Model file for the job. Use its own axes, mm. Face numbers are marked on the shaded views. Coordinates: 2 decimals unless noted, no trailing zeros. Write each loop counter-clockwise with the first axis right and the second up, starting at its lowest first coordinate (ties: lowest second). Pieces come first, ordered by that corner, then holes.
Q1. Band-saw the part on C-C, the plane z = 9.25. Write the cut outline in (x, y) (3 decimals).
Q2. Band-saw the part on B-B, the plane y = 25. Write the cut outline in (x, z).
Q3. Band-saw the part on A-A, the plane x = 0. Write the cut outline in (y, z) (3 decimals).
Q4. Drill centre lines: probe 1 along X at (y, z) = (0.5, 4.25); probe 2 along Y at (x, z) = (-23, 5.5); probe 3 along X at (y, z) = (-12, 0.75). Where is each one in solid material? Low to high.
Q5. Pin check, flat tips, straight feed: P1, Ø1, axis at x = -20.5, z = 3.5, coming from the -Y side; P2, Ø1.5, axis at x = -0.5, z = 7, coming from the -Y side; P3, Ø6, axis at x = -5, z = 6, coming from the -Y side. Stop position of each tip, or through.
Q6. Pull direction X, two halves, no side cores. Call the marked faces 1, 2 and 3: released by +X, released by -X, zero draft, split by the parting line, or undercut.
Q7. Band-saw the part on D-D, the plane z = 4.5. State how many separate pieces and enclosed holes the cut face has, plus the area to 3 significant figures.
from build123d import *

# Parameters (mm, degrees)
SKETCH1_R           = 30.5
SKETCH1_R_2         = 22.025
BOSS_EXTRUDE1_DEPTH = 3.5
LAPVSROTOR_START    = 3.5
SKETCH1_8_R         = 29.25
SKETCH1_8_R_2       = 22.025
LAPVSROTOR_DEPTH    = 10
CUT_EXTRUDE1_START  = 13.5
SKETCH1_9_R         = 1.55
CUT_EXTRUDE1_DEPTH  = 10
SKETCH2_R           = 22.05
SKETCH2_R_2         = 21
BOSS_EXTRUDE3_DEPTH = 1
SKETCH3_R           = 1.55
CUT_EXTRUDE2_DEPTH  = 46.196791922
CUT_EXTRUDE3_START  = 7.5
SKETCH4_R           = 28.075
SKETCH4_R_2         = 21
CUT_EXTRUDE3_DEPTH  = 6
SKETCH5_R           = 3
CUT_EXTRUDE4_DEPTH  = 2.5
CIRPATTERN1_COUNT   = 7


with BuildPart() as part:
    # Sketch1 → Boss-Extrude1 (new body)
    with BuildSketch(Plane.XY):
        Circle(SKETCH1_R)
        Circle(SKETCH1_R_2, mode=Mode.SUBTRACT)
    extrude(amount=BOSS_EXTRUDE1_DEPTH)

    # Sketch1<8> → lapvsrotor (add)
    with BuildSketch(Plane.XY.offset(LAPVSROTOR_START)):
        Circle(SKETCH1_8_R)
        Circle(SKETCH1_8_R_2, mode=Mode.SUBTRACT)
    extrude(amount=LAPVSROTOR_DEPTH)

    # Sketch1<9> → Cut-Extrude1 (cut)
    with BuildSketch(Plane.XY.offset(CUT_EXTRUDE1_START)):
        with Locations((0, 25)):
            Circle(SKETCH1_9_R)
        with Locations((10.847093478, 22.524221698)):
            Circle(SKETCH1_9_R)
        with Locations((19.545787062, 15.587245046)):
            Circle(SKETCH1_9_R)
        with Locations((24.373197805, 5.563023349)):
            Circle(SKETCH1_9_R)
        with Locations((24.373197805, -5.563023349)):
            Circle(SKETCH1_9_R)
        with Locations((19.545787062, -15.587245046)):
            Circle(SKETCH1_9_R)
        with Locations((10.847093478, -22.524221698)):
            Circle(SKETCH1_9_R)
        with Locations((0, -25)):
            Circle(SKETCH1_9_R)
        with Locations((-10.847093478, -22.524221698)):
            Circle(SKETCH1_9_R)
        with Locations((-19.545787062, -15.587245046)):
            Circle(SKETCH1_9_R)
        with Locations((-24.373197805, -5.563023349)):
            Circle(SKETCH1_9_R)
        with Locations((-24.373197805, 5.563023349)):
            Circle(SKETCH1_9_R)
        with Locations((-19.545787062, 15.587245046)):
            Circle(SKETCH1_9_R)
        with Locations((-10.847093478, 22.524221698)):
            Circle(SKETCH1_9_R)
    extrude(amount=-CUT_EXTRUDE1_DEPTH, mode=Mode.SUBTRACT)

    # Sketch2 → Boss-Extrude3 (add)
    with BuildSketch(Plane.XY):
        Circle(SKETCH2_R)
        Circle(SKETCH2_R_2, mode=Mode.SUBTRACT)
    extrude(amount=BOSS_EXTRUDE3_DEPTH)

    # Sketch3 → Cut-Extrude2 (cut, through all)
    with BuildSketch(Plane.XY):
        with Locations((5.89680475, 25.835589673)):
            Circle(SKETCH3_R)
        with Locations((23.875674999, 11.497919087)):
            Circle(SKETCH3_R)
        with Locations((23.875674999, -11.497919087)):
            Circle(SKETCH3_R)
        with Locations((5.89680475, -25.835589673)):
            Circle(SKETCH3_R)
        with Locations((-16.522479749, -20.718534285)):
            Circle(SKETCH3_R)
        with Locations((-26.5, 0)):
            Circle(SKETCH3_R)
        with Locations((-16.522479749, 20.718534285)):
            Circle(SKETCH3_R)
    extrude(amount=CUT_EXTRUDE2_DEPTH, mode=Mode.SUBTRACT)

    # Sketch4 → Cut-Extrude3 (cut)
    with BuildSketch(Plane.XY.offset(CUT_EXTRUDE3_START)):
        Circle(SKETCH4_R)
        Circle(SKETCH4_R_2, mode=Mode.SUBTRACT)
    extrude(amount=CUT_EXTRUDE3_DEPTH, mode=Mode.SUBTRACT)

    # Sketch5 → Cut-Extrude4 (cut)
    with BuildSketch(Plane.XY):
        with Locations((5.89680475, 25.835589673)):
            Circle(SKETCH5_R)
    cut_extrude4 = extrude(amount=CUT_EXTRUDE4_DEPTH, mode=Mode.SUBTRACT)

    # CirPattern1: Cut-Extrude4 ×7 about axis
    cirpattern1_axis = Axis((0, 0, 0), (0, 0, 1))
    for i in range(1, CIRPATTERN1_COUNT):
        add(cut_extrude4.rotate(cirpattern1_axis, i * 360 / CIRPATTERN1_COUNT), mode=Mode.SUBTRACT)


solid = part.part
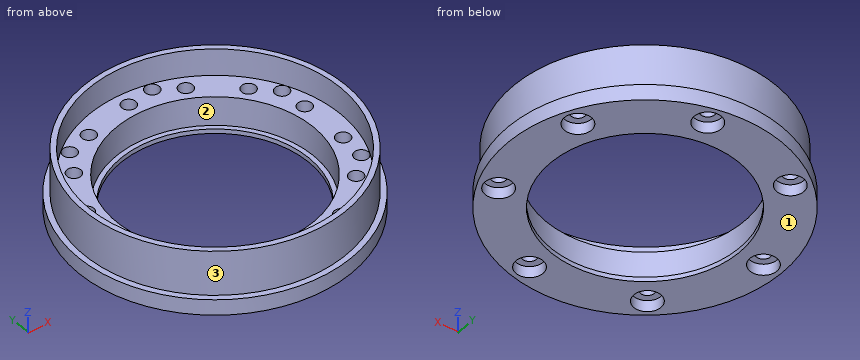
Answer sheet:
1. outline: circle Ø58.5 at (0, 0); hole circle Ø56.15 at (0, 0)
2. outline: (-17.47, 0) - (3.02, 0) - (3.02, 2.5) - (4.59, 2.5) - (4.59, 7.5) - (1.55, 7.5) - (1.55, 3.5) - (-1.55, 3.5) - (-1.55, 7.5) - (-12.78, 7.5) - (-12.78, 13.5) - (-15.18, 13.5) - (-15.18, 3.5) - (-17.47, 3.5) - close; (7.2, 2.5) - (8.78, 2.5) - (8.78, 0) - (17.47, 0) - (17.47, 3.5) - (15.18, 3.5) - (15.18, 13.5) - (12.78, 13.5) - (12.78, 7.5) - (7.2, 7.5) - close
3. outline: (-30.5, 0) - (-21, 0) - (-21, 1) - (-22.025, 1) - (-22.025, 7.5) - (-23.45, 7.5) - (-23.45, 3.5) - (-26.55, 3.5) - (-26.55, 7.5) - (-28.075, 7.5) - (-28.075, 13.5) - (-29.25, 13.5) - (-29.25, 3.5) - (-30.5, 3.5) - close; (21, 0) - (30.5, 0) - (30.5, 3.5) - (29.25, 3.5) - (29.25, 13.5) - (28.075, 13.5) - (28.075, 7.5) - (26.55, 7.5) - (26.55, 3.5) - (23.45, 3.5) - (23.45, 7.5) - (22.025, 7.5) - (22.025, 1) - (21, 1) - close
4. probe 1: x = -29.25 to -27.97, -25.03 to -22.02, 22.02 to 29.25
4. probe 2: y = -18.07 to -6.28, -4.84 to 4.84, 6.28 to 18.07
4. probe 3: x = -28.04 to -17.23, 17.23 to 20.92, 26.83 to 28.04
5. P1: stops at y = -23.03
5. P2: stops at y = -29.25
5. P3: stops at y = -30.32
6. face 1: zero draft
6. face 2: undercut
6. face 3: split by the parting line
7. separate pieces: 1
7. enclosed holes: 22
7. area: 1,010 mm2
